Source: CAD feature listing. Evaluate the final solid. Frame: model axes, mm. Give positions to 0.01 mm unless a question says otherwise; leave off trailing zeros. Order: outer loops, then holes, each group sorted by start corner. A loop starts at its lowest first (then second) coordinate and runs counter-clockwise, first axis right, second up. Notation, with made-up numbers: (14.25, -5.75) -> (45.25, -5.75) arc R25 ccw to (45.25, 28.25) -> close; hole circle Ø2 at (-12.5, 44.25). An arc over 180 degrees is marked (long way). Answer in a Markdown table with one row per item.
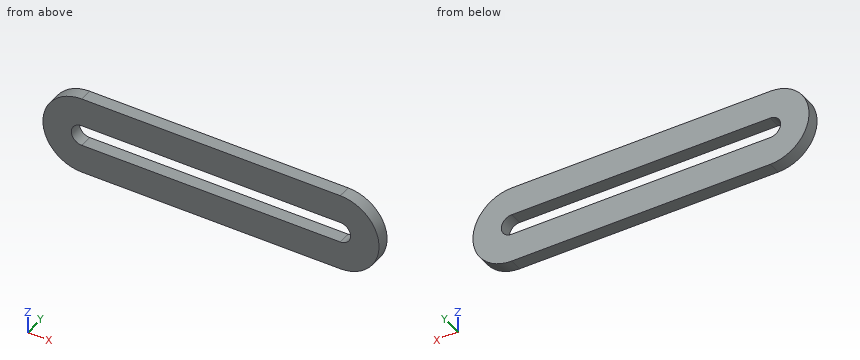
```python
from build123d import *

# Parameters (mm, degrees)
PAD_DEPTH = 2.5


with BuildPart() as part:
    # Sketch → Pad (new body)
    with BuildSketch(Plane.XZ):
        with BuildLine():
            ThreePointArc((0, 7.5), (-7.5, 0), (0, -7.5))
            Line((0, -7.5), (50, -7.5))
            ThreePointArc((50, -7.5), (57.5, 0), (50, 7.5))
            Line((50, 7.5), (0, 7.5))
        make_face()
        with BuildLine():
            ThreePointArc((0, 2), (-2, 0), (0, -2))
            Line((0, -2), (50, -2))
            ThreePointArc((50, -2), (52, 0), (50, 2))
            Line((50, 2), (0, 2))
        make_face(mode=Mode.SUBTRACT)
    extrude(amount=PAD_DEPTH)


solid = part.part
```
(1) Section query D-D (z = 4.5). Return the cut outline in (x, y).
A:
| item | result |
|---|---|
| outline | (-6, -2.5) -> (56, -2.5) -> (56, 0) -> (-6, 0) -> close |
(2) Section query B-B (y = -0.6). Return the cut outline in (x, z), plus the area to 3 significant figures.
A:
| item | result |
|---|---|
| outline | (0, -7.5) -> (50, -7.5) arc R7.5 ccw to (50, 7.5) -> (0, 7.5) arc R7.5 ccw to start; hole (0, -2) -> (50, -2) arc R2 ccw to (50, 2) -> (0, 2) arc R2 ccw to start |
| area | 714 mm^2 |
(3) Section query C-C (z = 0.5). Return the cut outline in (x, y), plus the area to 3 significant figures.
A:
| item | result |
|---|---|
| outline | (-7.48, -2.5) -> (-1.94, -2.5) -> (-1.94, 0) -> (-7.48, 0) -> close; (51.94, -2.5) -> (57.48, -2.5) -> (57.48, 0) -> (51.94, 0) -> close |
| area | 27.7 mm^2 |
(4) Section query A-A (x = 45). Return the cut outline in (y, z), plus the area to 3 significant figures.
A:
| item | result |
|---|---|
| outline | (-2.5, -7.5) -> (0, -7.5) -> (0, -2) -> (-2.5, -2) -> close; (-2.5, 2) -> (0, 2) -> (0, 7.5) -> (-2.5, 7.5) -> close |
| area | 27.5 mm^2 |
(5) Ray query, probe 1 along Z at (x, y) = (47, -1.1); probe 2 along X at (y, z) = (-1.8, 0.25); probe 3 along X at (y, z) = (-0.8, 0.5). Return the intervals inside material, ascending.
A:
| item | result |
|---|---|
| probe 1 | z = -7.5 to -2, 2 to 7.5 |
| probe 2 | x = -7.5 to -1.98, 51.98 to 57.5 |
| probe 3 | x = -7.48 to -1.94, 51.94 to 57.48 |
